```python
from build123d import *

# Parameters (mm, degrees)
F0_W     = 2057.4
F0_H     = 469.9
F0_W_2   = 2019.3
F0_H_2   = 431.8
F1_DEPTH = 479.425
F2_W     = 1981.2
F2_H     = 920.75
F3_DEPTH = 469.901
F4_W     = 431.8
F4_H     = 920.75
F5_DEPTH = 2057.401
F6_W     = 38.1
F6_H     = 38.1
F7_DEPTH = 38.1
F8_W     = 38.1
F8_H     = 38.1
F9_DEPTH = 381


with BuildPart() as f1:
    # F0 (on Top) → F1 (new body, symmetric)
    with BuildSketch(Plane.XY):
        Rectangle(F0_W, F0_H)
        Rectangle(F0_W_2, F0_H_2, mode=Mode.SUBTRACT)
    extrude(amount=F1_DEPTH, both=True)

    # F2 (on face) → F3 (cut, through all)
    with BuildSketch(Plane.XZ.offset(234.95)):
        with Locations((0, -19.05)):
            Rectangle(F2_W, F2_H)
    extrude(amount=-F3_DEPTH, mode=Mode.SUBTRACT)

    # F4 (on face) → F5 (cut, through all)
    with BuildSketch(Plane(origin=(-1028.7, 0, 0), x_dir=(0, -1, 0), z_dir=(-1, 0, 0))):
        with Locations((0, -19.05)):
            Rectangle(F4_W, F4_H)
    extrude(amount=-F5_DEPTH, mode=Mode.SUBTRACT)

    # F6 (on face) → F7 (join)
    with BuildSketch(Plane(origin=(0, 234.95, 0), x_dir=(-1, 0, 0), z_dir=(0, 1, 0))):
        with Locations((0, 460.375)):
            Rectangle(F6_W, F6_H)
    extrude(amount=F7_DEPTH)

    # F8 (on face) → F9 (join)
    with BuildSketch(Plane.XY.offset(479.425)):
        with Locations((0, 254)):
            Rectangle(F8_W, F8_H)
    extrude(amount=F9_DEPTH)


solid = f1.part
```
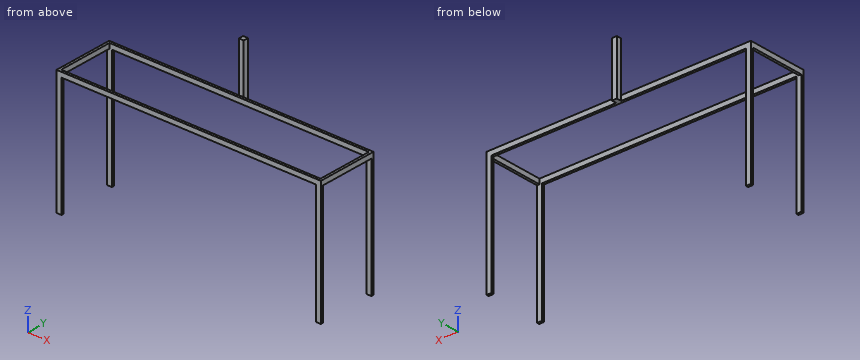
Can you work these out from the model? Positions are in its coordinate system, mm. Give positions to 0.01 mm unless a question says otherwise; leave off trailing zeros. Loops run counter-clockwise (first coordinate to the right, second up) from the corner with the lowest first, then second, coordinate; pieces in that order, holes last. Notation, with made-up numbers: M 27.25,-38 L 50.25,-38 A9 ccw 50.25,-28 Z; hole C 61,-15 d6. An arc over 180 degrees is marked long. Answer in a Markdown table with one row per item.
1. Suppose I cut it at B-B on x = -569.5. Write out the boundary of the cut face in (y, z) (3 decimals), plus the area to 3 significant figures.
Taken from the geometry:
| item | result |
|---|---|
| outline | M -234.95,441.325 L -215.9,441.325 L -215.9,479.425 L -234.95,479.425 Z; M 215.9,441.325 L 234.95,441.325 L 234.95,479.425 L 215.9,479.425 Z |
| area | 1,450 mm² |
2. Suppose I cut it at C-C on y = 187. Write out the boundary of the cut face in (x, z) (3 decimals), plus the area to 3 significant figures.
Taken from the geometry:
| item | result |
|---|---|
| outline | M -1028.7,441.325 L -1009.65,441.325 L -1009.65,479.425 L -1028.7,479.425 Z; M 1009.65,441.325 L 1028.7,441.325 L 1028.7,479.425 L 1009.65,479.425 Z |
| area | 1,450 mm² |
3. For pin 1 Ø11.5 at (y, z) = (258, 563.5) entering from +X; pin 2 Ø5.5 at (x, y) = (1020.5, -71) entering from -Z (3 decimals), each with a flat end and sliding along its axis, tell me the tip position at first contact or that it passes through.
Taken from the geometry:
| item | result |
|---|---|
| pin 1 | stops at x = 19.05 |
| pin 2 | stops at z = 441.325 |
4. Suppose I cut it at A-A on z = -131.5. Write out the boundary of the cut face in (x, y).
Taken from the geometry:
| item | result |
|---|---|
| outline | M -1028.7,-234.95 L -990.6,-234.95 L -990.6,-215.9 L -1028.7,-215.9 Z; M -1028.7,215.9 L -990.6,215.9 L -990.6,234.95 L -1028.7,234.95 Z; M 990.6,-234.95 L 1028.7,-234.95 L 1028.7,-215.9 L 990.6,-215.9 Z; M 990.6,215.9 L 1028.7,215.9 L 1028.7,234.95 L 990.6,234.95 Z |
